Can you work these out from the drawing? Everything is in mm from the part's minimum corner. Round coordinates to 2 decimals unless told otherwise and drop trailing zeros. Write each loop counter-clockwise with the first axis right and the second up, starting at its lowest first coordinate (ties: lowest second). Pieces come first, ordered by that corner, then holes. Notation, with made-up numbers: (-20, -37) -> (1, -37) arc R11 cw to (1, -20) -> close; hole circle Ø7 at (34.5, 76.5). An arc over 180 degrees is marked (long way). One line per question, with ' | ' between items. Start each with the question number.
1. If I drill on line 1 along Z through (x, y) = (24.5, 22); line 2 along X through (y, z) = (36, 8); line 3 along X through (y, z) = (33.5, 39.5), over which ranges is the centre line in solid material (lowest first)? Write a range as [from, to].
2. Thinking about a two-plate mould opening in Z: for the marked faces 1, 2 and 3, which applies, released by +Z, released by -Z, zero draft, split by the parting line, or undercut?
3. Imagine slicing it at A-A, the plane z = 22. List the corners of the cut face in (x, y) for me, and give its area (3 significant figures).
4. Imagine slicing it at C-C, the plane y = 4.5. List the corners of the cut face in (x, z) for me.
5. Imagine slicing it at D-D, the plane z = 12. List the corners of the cut face in (x, y) for me.
6. For pin 1 Ø8 at (x, y) = (21.5, 16) entering from +Z; pin 2 Ø1 at (x, y) = (11.5, 32) entering from +Z; pin 3 Ø6 at (y, z) = (32.5, 9.5) entering from -X, each with a flat end and sliding along its axis, tell me the tip position at first contact or that it passes through.
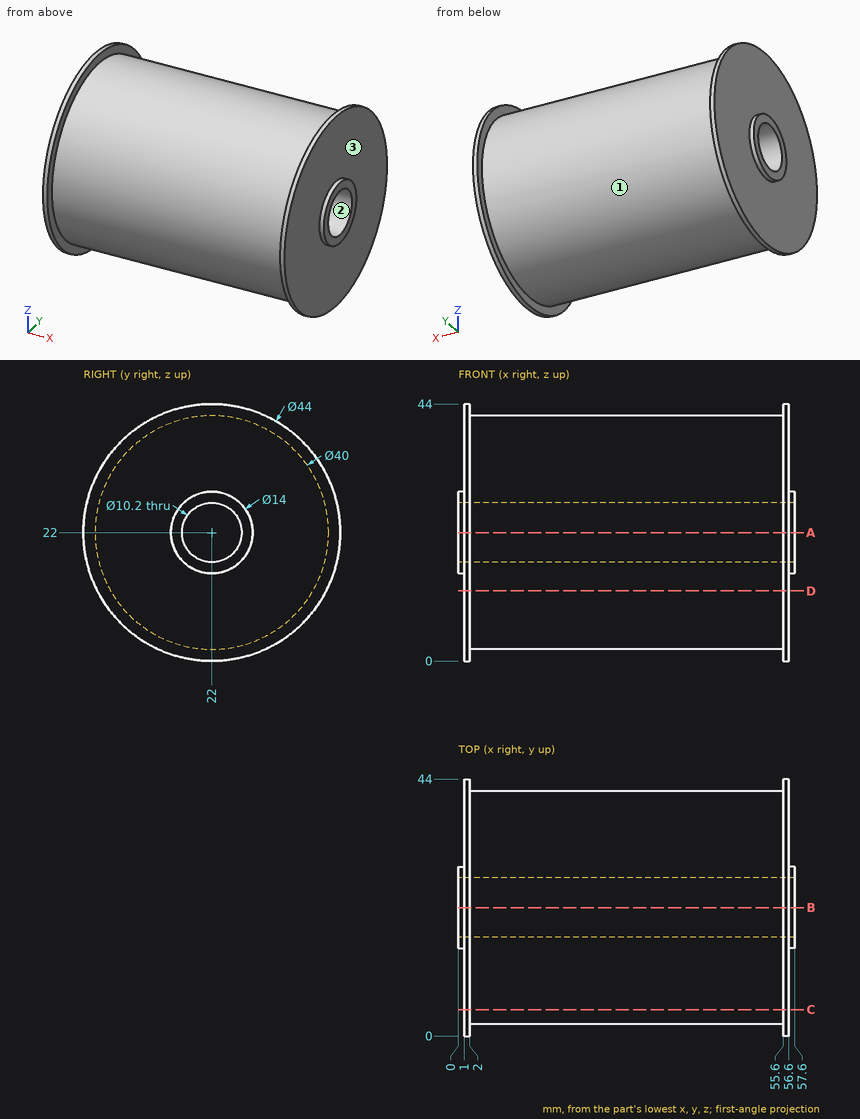
Geometry results:
1) line 1: z = [2, 16.9], [27.1, 42] | line 2: x = [1, 56.6] | line 3: x = [1, 2], [55.6, 56.6]
2) face 1: split by the parting line | face 2: undercut | face 3: zero draft
3) outline: (0, 15) -> (1, 15) -> (1, 0) -> (2, 0) -> (2, 2) -> (55.6, 2) -> (55.6, 0) -> (56.6, 0) -> (56.6, 15) -> (57.6, 15) -> (57.6, 16.9) -> (0, 16.9) -> close; (0, 27.1) -> (57.6, 27.1) -> (57.6, 29) -> (56.6, 29) -> (56.6, 44) -> (55.6, 44) -> (55.6, 42) -> (2, 42) -> (2, 44) -> (1, 44) -> (1, 29) -> (0, 29) -> close | area: 1,670 mm2
4) outline: (1, 8.67) -> (2, 8.67) -> (2, 12.32) -> (55.6, 12.32) -> (55.6, 8.67) -> (56.6, 8.67) -> (56.6, 35.33) -> (55.6, 35.33) -> (55.6, 31.68) -> (2, 31.68) -> (2, 35.33) -> (1, 35.33) -> close
5) outline: (1, 2.4) -> (2, 2.4) -> (2, 4.68) -> (55.6, 4.68) -> (55.6, 2.4) -> (56.6, 2.4) -> (56.6, 41.6) -> (55.6, 41.6) -> (55.6, 39.32) -> (2, 39.32) -> (2, 41.6) -> (1, 41.6) -> close
6) pin 1: stops at z = 41.9 | pin 2: stops at z = 39.6 | pin 3: stops at x = 1
